Source: CAD feature listing. Evaluate the final solid. Frame: model axes, mm. A direction names the side the tool comes from. Give positions to 0.01 mm unless a question says otherwise; leave off trailing zeros. Order: outer loops, then holes, each group sorted by start corner. A loop starts at its lowest first (then second) coordinate and runs counter-clockwise, first axis right, second up. Notation, with made-up numbers: M 59,7.25 L 79,7.25 A18 ccw 79,37.25 Z; hole C -0.5,5 d7. An arc over 180 degrees is marked long. Answer as a JSON object with one key per item and string values. Group by question number.
1. Section query D-D (x = 14.5). Output: boundary loops of the cut face in (y, z).
2. Set-up query: faces 4 (the flat face through (1.1, -12.1, 4)), 5 (the cylindrical face through (-12.704, -6.219, 4.056)). Return all of +Z, -Z, +X, -X, +Y, -Y with unobstructed straight access to the full face (end or side cutting, diameter ignored); none if empty.
3. Section query C-C (y = -4). Output: boundary loops of the cut face in (x, z).
4. Pin query (flat end, axial travel): P1, Ø1.5, axis at y = 9, z = 3, coming from the -X side; P2, Ø2, axis at y = -11, z = 2, coming from the +X side; P3, Ø3, axis at x = 11, y = 0, coming from the +Z side. Return the tip coordinate at first contact, or that it passes through.
5. Pull-direction query (X, two-part tool) for faces 1 (the flat face through (-4, -4, 0)), 2 (the cylindrical face through (-13.887, 10.648, 3.944)), 3 (the cylindrical face through (-0.54, -13.44, 6.03)); classes: +X half, -X half, draft (parallel to the pull), parting line (faces both ways), or undercut.
6. Section query A-A (x = 0). Output: boundary loops of the cut face in (y, z).
7. Material intervals for L1, parallel to Y at x = 0, z = 3; L2, parallel to X at y = 2, z = 4.75; L3, parallel to X at y = -6, z = 6, sorted ascending. Write a range as [from, to].
Autodesk Inventor part; units mm, degrees
ref_plane "YZ Plane" through (0, 0, 0) normal (1, 0, 0) x (0, 1, 0)
ref_plane "XZ Plane" through (0, 0, 0) normal (0, 1, 0) x (-1, 0, 0)
ref_plane "XY Plane" through (0, 0, 0) normal (0, 0, 1) x (1, 0, 0)
sketch "스케치3" plane through (0, 0, 0) normal (0, 0, 1) x (1, 0, 0)
  circle A0 centre (0, 0) radius 5.2
  circle A1 centre (0, 0) radius 17.5
  dimension "d13" = 10.4
  dimension "d14" = 35
extrude "돌출3" add sketch "스케치3" along normal blind 8
sketch "스케치4" plane through (0, 0, 8) normal (0, 0, 1) x (1, 0, 0)
  circle A0 centre (0, 0) radius 11
  line L0 (0, 0) -> (0, 11)
  line L1 (0, 0) -> (11, 0) construction
  circle A1 centre (0, 11) radius 1.35
  circle A2 centre (-7.7782, 7.7782) radius 1.35
  circle A3 centre (-11, 0) radius 1.35
  circle A4 centre (-7.7782, -7.7782) radius 1.35
  circle A5 centre (0, -11) radius 1.35
  circle A6 centre (7.7782, -7.7782) radius 1.35
  circle A7 centre (11, 0) radius 1.35
  circle A8 centre (7.7782, 7.7782) radius 1.35
  dimension "d17" = 22
  dimension "d18" = 11
  dimension "d19" = 90
  dimension "d20" = 2.7
  dimension "d23" = 360
extrude "돌출4" cut sketch "스케치4" against normal up to surface (8 mm away) contours A0 A7 | A0 A7 | A8 A0 | A0 A8 | A6 A0 | A0 A6 | A1 L0 A0 | A0 A1 | A5 A0 | A0 A5 | L0 A1 A0 | A4 A0 | A0 A4 | A2 A0 | A0 A2 | A3 A0 | A0 A3
sketch "스케치5" plane through (0, 0, 8) normal (0, 0, 1) x (1, 0, 0)
  circle A0 centre (7.7782, 7.7782) radius 1.35
  circle A1 centre (11, 0) radius 1.35
  circle A2 centre (0, -11) radius 1.35
  circle A3 centre (-11, 0) radius 1.35
  circle A4 centre (0, 11) radius 1.35
  circle A5 centre (-7.7782, 7.7782) radius 1.35
  circle A6 centre (-7.7782, -7.7782) radius 1.35
  circle A7 centre (7.7782, -7.7782) radius 1.35
  circle A8 centre (0, 0) radius 5.2
  circle A9 centre (0, 0) radius 17.5
  circle A10 centre (-11, 0) radius 2.5
  circle A11 centre (-7.7782, 7.7782) radius 2.5
  circle A12 centre (0, 11) radius 2.5
  circle A13 centre (7.7782, 7.7782) radius 2.5
  circle A14 centre (11, 0) radius 2.5
  circle A15 centre (7.7782, -7.7782) radius 2.5
  circle A16 centre (0, -11) radius 2.5
  circle A17 centre (-7.7782, -7.7782) radius 2.5
  dimension "d27" = 5
  dimension "d28" = 5
  dimension "d29" = 5
  dimension "d30" = 5
  dimension "d31" = 5
  dimension "d32" = 5
  dimension "d33" = 5
  dimension "d34" = 5
extrude "돌출5" cut sketch "스케치5" against normal blind 4 contours A10 | A11 | A12 | A13 | A14 | A15 | A16 | A17
sketch "스케치6" plane through (0, 0, 8) normal (0, 0, 1) x (1, 0, 0)
  circle A0 centre (0, 0) radius 14
  line L0 (0, 0) -> (-5.7403, 13.8582)
  line L1 (0, 0) -> (15, 0) construction
  circle A1 centre (-5.7403, 13.8582) radius 1.25
  circle A2 centre (-13.8582, 5.7403) radius 1.25
  circle A3 centre (-13.8582, -5.7403) radius 1.25
  circle A4 centre (-5.7403, -13.8582) radius 1.25
  circle A5 centre (5.7403, -13.8582) radius 1.25
  circle A6 centre (13.8582, -5.7403) radius 1.25
  circle A7 centre (13.8582, 5.7403) radius 1.25
  circle A8 centre (5.7403, 13.8582) radius 1.25
  dimension "d37" = 28
  dimension "d38" = 15
  dimension "d39" = 112.5
  dimension "d40" = 2.5
  dimension "d43" = 360
extrude "돌출6" cut sketch "스케치6" against normal up to surface (8 mm away) contours A7 A0 | A0 A7 | A6 A0 | A0 A6 | A8 A0 | A0 A8 | A5 A0 | A0 A5 | A1 L0 A0 | A0 A1 | A4 A0 | A0 A4 | L0 A1 A0 | A3 A0 | A0 A3 | A2 A0 | A0 A2
properties part number "조인트4베어링관절혼" material "알루미늄 6061"
Answer sheet:
{
 "1": {"outline": "M -9.8,0 L -6.81,0 L -6.81,8 L -9.8,8 Z; M -4.67,0 L 4.67,0 L 4.67,8 L -4.67,8 Z; M 6.81,0 L 9.8,0 L 9.8,8 L 6.81,8 Z"},
 "2": {"face 4": "+Z", "face 5": "+Z, -Z"},
 "3": {"outline": "M -17.04,0 L -3.32,0 L -3.32,8 L -17.04,8 Z; M 3.32,0 L 17.04,0 L 17.04,8 L 3.32,8 Z"},
 "4": {"P1": "x = -15.43", "P2": "x = 14.36", "P3": "z = 4"},
 "5": {"face 1": "draft", "face 2": "parting line", "face 3": "undercut"},
 "6": {"outline": "M -17.5,0 L -12.35,0 L -12.35,4 L -13.5,4 L -13.5,8 L -17.5,8 Z; M -9.65,0 L -5.2,0 L -5.2,8 L -8.5,8 L -8.5,4 L -9.65,4 Z; M 5.2,0 L 9.65,0 L 9.65,4 L 8.5,4 L 8.5,8 L 5.2,8 Z; M 12.35,0 L 17.5,0 L 17.5,8 L 13.5,8 L 13.5,4 L 12.35,4 Z"},
 "7": {"L1": "[-17.5, -12.35], [-9.65, -5.2], [5.2, 9.65], [12.35, 17.5]", "L2": "[-17.39, -12.5], [-9.5, -4.8], [4.8, 9.5], [12.5, 17.39]", "L3": "[-16.44, -15.08], [-12.64, -9.54], [-6.02, 6.02], [9.54, 12.64], [15.08, 16.44]"}
}
